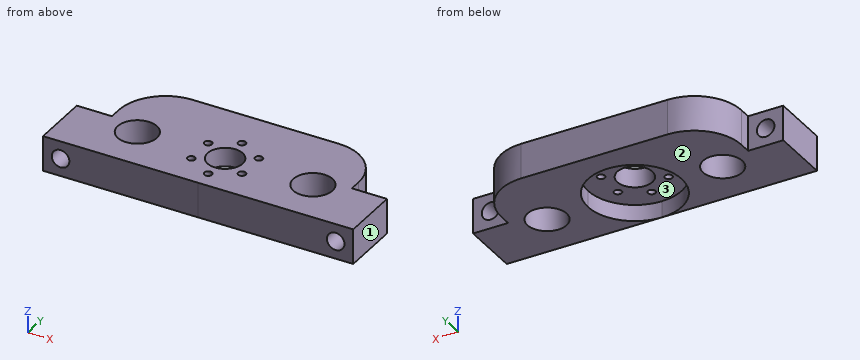
Autodesk Inventor part; units mm, degrees
ref_plane "Work Plane2" through (-26.5, 15, 0) normal (0, 1, 0) x (1, 0, 0)
ref_plane "YZ Plane" through (0, 0, 0) normal (1, 0, 0) x (0, 1, 0)
ref_plane "XZ Plane" through (0, 0, 0) normal (0, 1, 0) x (-1, 0, 0)
sketch "Sketch1" plane through (0, 0, 0) normal (0, 0, 1) x (1, 0, 0)
  line L0 (-23.75, 0) -> (0, 0)
  circle A0 centre (0, 8) radius 8
  line L1 (0, 0) -> (23.75, 0)
  line L2 (12.5, 20) -> (-12.5, 20)
  circle A1 centre (15, 8) radius 3.35
  circle A2 centre (-15, 8) radius 3.35
  circle A3 centre (0, 8) radius 3
  line L3 (-23.75, 0) -> (-26.5, 0)
  line L4 (23.75, 0) -> (26.5, 0)
  line L5 (-26.5, 0) -> (-20.5, 0)
  line L6 (-20.5, 10) -> (-26.5, 10)
  line L7 (-26.5, 10) -> (-26.5, 0)
  line L8 (-20.5, 10) -> (-20.5, 12)
  line L9 (26.5, 0) -> (20.5, 0)
  line L10 (20.5, 10) -> (26.5, 10)
  line L11 (26.5, 10) -> (26.5, 0)
  line L12 (20.5, 10) -> (20.5, 12)
  arc A4 (-12.5, 20) -> (-20.5, 12) centre (-12.5, 12) ccw
  arc A5 (20.5, 12) -> (12.5, 20) centre (12.5, 12) ccw
  point P0 (20.5, 20)
  point P1 (-20.5, 20)
  dimension "d0" = 15
  dimension "d1" = 15
  dimension "d8" = 12
  dimension "d9" = 12
  dimension "d10" = 12
  dimension "d11" = 8
  dimension "d17" = 6.7
  dimension "d18" = 6.7
  dimension "d21" = 6
  dimension "d22" = 6
  dimension "d23" = 10
  dimension "d24" = 10
  dimension "d36" = 41
  dimension "d37" = 8
  dimension "d38" = 20
  dimension "d39" = 26.5
  dimension "d40" = 8
ref_plane "Work Plane2" through (-26.5, 15, 0) normal (0, 1, 0) x (1, 0, 0)
sketch "Sketch2" plane through (-26.5, 15, 0) normal (0, 1, 0) x (1, 0, 0)
  line L0 (0, 0) -> (6, 0)
  line L1 (0, 0) -> (0, -6)
  line L2 (6, -6) -> (0, -6)
  line L3 (6, 0) -> (6, -6)
  line L4 (47, 0) -> (53, 0)
  line L5 (47, 0) -> (47, -6)
  line L6 (53, -6) -> (47, -6)
  line L7 (53, 0) -> (53, -6)
  circle A0 centre (3, -3) radius 1.5
  circle A1 centre (50, -3) radius 1.5
  point P0 (26.5, 0)
  dimension "d27" = 3
  dimension "d28" = 3
extrude "Extrusion3" add sketch "Sketch1" along normal blind 6 contours L3 L7 L6 L8 A4 L2 A5 L12 L10 L11 L4 L1 L0
hole "Hole2" at (-23.5, 15, 3) at (23.5, 15, 3) direction (0, -1, 0) diameter 3 end through all
sketch "Sketch3" plane through (0, 0, 6) normal (0, 0, 1) x (1, 0, 0)
  circle A0 centre (0, 8) radius 8
  circle A1 centre (0, 13) radius 0.65
  circle A2 centre (-4.3301, 10.5) radius 0.65
  circle A3 centre (-4.3301, 5.5) radius 0.65
  circle A4 centre (0, 3) radius 0.65
  circle A5 centre (4.3301, 5.5) radius 0.65
  circle A6 centre (4.3301, 10.5) radius 0.65
  circle A7 centre (0, 8) radius 3
  point P0 (0, 0)
  dimension "d53" = 1.3
  dimension "d56" = 360
  dimension "d60" = 6
extrude "Extrusion6" add sketch "Sketch3" against normal blind 3.2
properties part number "Base_Motor_acrilico_15"
Check sheet for the modelled part. Datum: model origin and axes. Units: mm. Face numbers are marked on the shaded views. Give positions to 0.01 mm unless a question says otherwise; leave off trailing zeros. Write each loop counter-clockwise with the first axis right and the second up, starting at its lowest first coordinate (ties: lowest second). Pieces come first, ordered by that corner, then holes. Notation, with made-up numbers: (-16.5, -5) -> (12.5, -5) arc R27 ccw to (12.5, 21) -> close; hole circle Ø10 at (86.25, 38.25). An arc over 180 degrees is marked (long way). Use one line per item in the form item = value. Start each with the question number.
1. Section check A-A (z = 3.6). Count the separate pieces of the cut face and the enclosed holes in it, and give its area (3 significant figures).
2. Go/stop test with flat-tipped pins: P1, Ø8, axis at x = 0, y = 8, coming from the -Z side; P2, Ø3, axis at y = 18, z = 2, coming from the +X side; P3, Ø1.6, axis at y = 11, z = 2.5, coming from the -X side. Record where each tip stops, or that it passes through.
3. Section check B-B (x = 23.5). Record the cut outline in (y, z), and give its area (3 significant figures).
4. Mould release check, pull along X, two halves, no side actions. Record for the marked faces 1, 2 and 3: pulls with the +X half, pulls with the -X half, needs draft (parallel to the pull), parting line crosses it, or undercut.
5. Thickness scan on line 1 along Y through (x, z) = (0, 3.95); line 2 along X through (y, z) = (11, 2.2); line 3 along X through (y, z) = (2.5, 3). Record the ranges inside material, lowest first. Write a range as from..to.
6. Section check D-D (y = 9). Record the cut outline in (x, z), and give its area (3 significant figures).
Conclusion:
q1.separate_pieces = 3
q1.enclosed_holes = 9
q1.area = 751 mm²
q2.P1 = 2.8
q2.P2 = 19.11
q2.P3 = -20.5
q3.outline = (0, 0) -> (10, 0) -> (10, 1.5) -> (0, 1.5) -> close; (0, 4.5) -> (10, 4.5) -> (10, 6) -> (0, 6) -> close
q3.area = 30.0 mm²
q4.face_1 = pulls with the +X half
q4.face_2 = needs draft
q4.face_3 = undercut
q5.line_1 = 0..2.35, 3.65..5, 11..12.35, 13.65..20
q5.line_2 = -20.5..-16.49, -13.51..-7.42, 7.42..13.51, 16.49..20.5
q5.line_3 = -26.5..-25, -22..-0.42, 0.42..22, 25..26.5
q6.outline = (-26.5, 0) -> (-18.2, 0) -> (-18.2, 6) -> (-26.5, 6) -> close; (-11.8, 0) -> (-7.94, 0) -> (-7.94, 2.8) -> (-2.83, 2.8) -> (-2.83, 6) -> (-11.8, 6) -> close; (2.83, 2.8) -> (7.94, 2.8) -> (7.94, 0) -> (11.8, 0) -> (11.8, 6) -> (2.83, 6) -> close; (18.2, 0) -> (26.5, 0) -> (26.5, 6) -> (18.2, 6) -> close; hole circle Ø3 at (-23.5, 3); hole circle Ø3 at (23.5, 3)
q6.area = 165 mm²
